Autodesk Inventor part; units mm, degrees
ref_plane "YZ Plane" through (0, 0, 0) normal (1, 0, 0) x (0, 1, 0)
ref_plane "XZ Plane" through (0, 0, 0) normal (0, 1, 0) x (-1, 0, 0)
ref_plane "XY Plane" through (0, 0, 0) normal (0, 0, 1) x (1, 0, 0)
sketch "Szkic1" plane through (0, 0, 0) normal (0, 1, 0) x (-1, 0, 0)
  line L0 (0, 0) -> (-100, 0)
  line L1 (-100, 0) -> (-100, -40)
  line L2 (-100, -40) -> (0, -40)
  line L3 (0, -40) -> (0, 0)
  dimension "d0" = 100
  dimension "d1" = 40
extrude "Wyciągnięcie proste1" add sketch "Szkic1" along normal blind 5
sketch "Szkic4" plane through (100, 0, 0) normal (1, 0, 0) x (0, 0, -1)
  line L0 (0, 5) -> (40, 5)
  line L1 (0, 5) -> (4.346, 0)
  line L2 (0, 0) -> (40, 0)
  line L3 (0, 0) -> (0, 5)
  line L4 (0, 0) -> (0, 5)
  line L5 (0, 5) -> (4.346, 0)
extrude "Wyciągnięcie proste2" cut sketch "Szkic4" against normal blind 100
sketch "Szkic5" plane through (100, 0, -40) normal (1, 0, 0) x (0, 0, -1)
  line L0 (-40, 5) -> (0, 5)
  line L1 (-40, 5) -> (-35, 0)
  line L2 (-35.654, 0) -> (0, 0)
  line L3 (-40, 5) -> (-32.9289, 5) construction
  line L4 (-35, 0) -> (-40, 0)
  line L5 (-35.654, 0) -> (-40, 5)
  line L6 (-40, 0) -> (-40, 5)
  dimension "d6" = 45
extrude "Wyciągnięcie proste3" cut sketch "Szkic5" against normal blind 100.25
sketch "Szkic6" plane through (100, 0, -40) normal (1, 0, 0) x (0, 0, -1)
  line L0 (0, 5) -> (-40, 5)
  line L1 (-40, 5) -> (-38, 5)
  line L2 (-38, 5) -> (-33, 0)
  line L3 (0, 0) -> (-35, 0)
  line L4 (-33, 0) -> (-35, 0)
  line L5 (-35, 0) -> (-40, 5)
  point P0 (-40, 0)
  dimension "d9" = 2
  dimension "d10" = 135
extrude "Wyciągnięcie proste4" cut sketch "Szkic6" against normal blind 100.25
sketch "Szkic7" plane through (100, 0, -40) normal (1, 0, 0) x (0, 0, -1)
  line L0 (-33, 0) -> (-38, 5)
  line L1 (-38, 5) -> (-36, 5)
  line L2 (0, 5) -> (-38, 5)
  line L3 (-36, 5) -> (-31, 0)
  line L4 (0, 0) -> (-33, 0)
  line L5 (-31, 0) -> (-33, 0)
  line L6 (-33, 0) -> (-38, 5)
  point P0 (-40, 0)
  dimension "d13" = 2
  dimension "d14" = 135
extrude "Wyciągnięcie proste5" cut sketch "Szkic7" against normal blind 100
sketch "Szkic13" plane through (0, 5, 0) normal (0, 1, 0) x (1, 0, 0)
  line L0 (16, 12) -> (28, 12)
  line L1 (28, 12) -> (28, 24)
  line L2 (28, 24) -> (16, 24)
  line L3 (16, 24) -> (16, 12)
  point P0 (0, 0)
  dimension "d17" = 12
  dimension "d18" = 12
extrude "Wyciągnięcie proste6" cut sketch "Szkic13" against normal blind 10
sketch "Szkic14" plane through (0, 5, 0) normal (0, 1, 0) x (1, 0, 0)
  line L0 (84, 12) -> (72, 12)
  line L1 (72, 12) -> (72, 24)
  line L2 (72, 24) -> (84, 24)
  line L3 (84, 24) -> (84, 12)
  point P0 (0, 0)
  dimension "d21" = 12
  dimension "d22" = 12
extrude "Wyciągnięcie proste7" cut sketch "Szkic14" against normal blind 10
properties part number "Helenowiak_plug"
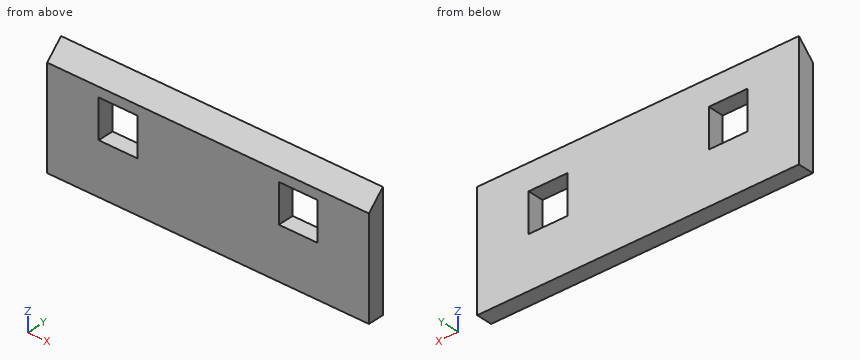
Part model, mm, in its own coordinate system. Round coordinates to 2 decimals unless told otherwise and drop trailing zeros. Write each loop counter-clockwise with the first axis right and the second up, starting at its lowest first coordinate (ties: lowest second). Pieces come first, ordered by that corner, then holes. Notation, with made-up numbers: (68, 10.25) -> (120, 10.25) arc R12 cw to (120, 15.25) -> close; hole circle Ø2 at (78, -17.5). An arc over 180 degrees is marked (long way). Return JSON: item names as keys, results as strings. Group by question number.
Q1. Probe L1, parallel to X at y = 2, z = -15.5; L2, parallel to Z at x = 26, y = 3.6; L3, parallel to Z at x = 18, y = 0.35. List the from-to ranges inside material, lowest first. Write a range as [from, to].
Q2. Saw through at D-D on z = -6.5. Write the cut outline in (x, y).
Q3. Saw through at B-B on y = 2.55. Write the cut outline in (x, z).
Q4. Saw through at A-A on x = 17.5. Write the cut outline in (y, z), plus the area to 4 significant figures.
Q5. Saw through at C-C on z = -16.5. Write the cut outline in (x, y).
Q6. Pin check, flat tip, straight feed: pin 1 (1.5 mm diameter, centred on x = 39.5, y = 2.5, fed in from +Z). Stop position of the tip, or through.
Answer:
{
 "1": {"L1": "[0, 16], [28, 72], [84, 100]", "L2": "[-40, -24], [-12, -5.4]", "L3": "[-40, -24], [-12, -8.65]"},
 "2": {"outline": "(0, 2.5) -> (100, 2.5) -> (100, 5) -> (0, 5) -> close"},
 "3": {"outline": "(0, -40) -> (100, -40) -> (100, -6.45) -> (0, -6.45) -> close; hole (16, -24) -> (28, -24) -> (28, -12) -> (16, -12) -> close; hole (72, -24) -> (84, -24) -> (84, -12) -> (72, -12) -> close"},
 "4": {"outline": "(0, -40) -> (5, -40) -> (5, -24) -> (0, -24) -> close; (0, -12) -> (5, -12) -> (5, -4) -> (0, -9) -> close", "area": "107.5 mm2"},
 "5": {"outline": "(0, 0) -> (16, 0) -> (16, 5) -> (0, 5) -> close; (28, 0) -> (72, 0) -> (72, 5) -> (28, 5) -> close; (84, 0) -> (100, 0) -> (100, 5) -> (84, 5) -> close"},
 "6": {"pin 1": "z = -5.75"}
}
